```python
from build123d import *

# Parameters (mm, degrees)
SKETCH1_W           = 25.4
SKETCH1_H           = 12.7
BOSS_EXTRUDE1_DEPTH = 3.175
SKETCH2_W           = 6.4262
SKETCH2_H           = 3.175
BOSS_EXTRUDE2_DEPTH = 3.175
CUT_EXTRUDE1_DEPTH  = 3.175


with BuildPart() as part:
    # Sketch1 → Boss-Extrude1 (new body)
    with BuildSketch(Plane(origin=(0, 0, 0), x_dir=(1, 0, 0), z_dir=(0, 1, 0))):
        Rectangle(SKETCH1_W, SKETCH1_H)
    extrude(amount=BOSS_EXTRUDE1_DEPTH)

    # Sketch2 → Boss-Extrude2 (add)
    with BuildSketch(Plane.XY.offset(6.35)):
        with Locations((9.4869, 1.5875)):
            Rectangle(SKETCH2_W, SKETCH2_H)
        with Locations((-3.2893, 1.5875)):
            Rectangle(SKETCH2_W, SKETCH2_H)
    boss_extrude2 = extrude(amount=BOSS_EXTRUDE2_DEPTH)

    # Mirror1: Boss-Extrude2 across plane
    add(boss_extrude2.mirror(Plane.XY))

    # Sketch3 → Cut-Extrude1 (cut)
    with BuildSketch(Plane(origin=(0, 3.175, 0), x_dir=(1, 0, 0), z_dir=(0, 1, 0))):
        Polygon((-6.5024, -6.35), (-12.7, 6.35), (-12.7, -6.35), align=None)
    extrude(amount=-CUT_EXTRUDE1_DEPTH, mode=Mode.SUBTRACT)


solid = part.part
```
Design review of the part built by this model. Coordinates are the model's own, in mm. A direction names the side the tool comes from. Coordinates: 2 decimals unless noted, no trailing zeros. Order: outer loops, then holes, each group sorted by start corner. A loop starts at its lowest first (then second) coordinate and runs counter-clockwise, first axis right, second up. Notation, with made-up numbers: (-4.5, 63.5) - (5.5, 63.5) arc R27 ccw to (5.5, 98.5) - close; hole circle Ø7 at (73, -37). An arc over 180 degrees is marked (long way). Answer in a Markdown table with one row per item.
(1) Consider section C-C on z = -0.75. State the section outline as (x, y) points (3 decimals), plus the area to 3 significant figures.
Checked values:
| item | result |
|---|---|
| outline | (-9.967, 0) - (12.7, 0) - (12.7, 3.175) - (-9.967, 3.175) - close |
| area | 72.0 mm^2 |
(2) Consider section A-A on z = -7.25. State the section outline as (x, y) points (3 decimals), plus the area to 3 significant figures.
Checked values:
| item | result |
|---|---|
| outline | (-6.502, 0) - (-0.076, 0) - (-0.076, 3.175) - (-6.502, 3.175) - close; (6.274, 0) - (12.7, 0) - (12.7, 3.175) - (6.274, 3.175) - close |
| area | 40.8 mm^2 |
(3) Consider section B-B on y = 2.8. State the section outline as (x, z) points (3 decimals), plus the area to 3 significant figures.
Checked values:
| item | result |
|---|---|
| outline | (-12.7, -6.35) - (-6.502, -6.35) - (-6.502, -9.525) - (-0.076, -9.525) - (-0.076, -6.35) - (6.274, -6.35) - (6.274, -9.525) - (12.7, -9.525) - (12.7, 9.525) - (6.274, 9.525) - (6.274, 6.35) - (-0.076, 6.35) - (-0.076, 9.525) - (-6.502, 9.525) - (-6.502, 6.35) - close |
| area | 365 mm^2 |
(4) For faces 4 (the flat face through (3, 0, 0)), 5 (the flat face through (6.274, 2, -8)), 6 (the flat face through (-0.076, 2, 8)), 7 (the flat face through (-6.502, 2, -8)), list the 3-axis set-ups (+Z, -Z, +X, -X, +Y, -Y) from which the entire face can be reached by the end or side of a thin tool; tool diameter is ignored.
Checked values:
| item | result |
|---|---|
| face 4 | +Z, -Z, +X, -X, -Y |
| face 5 | -Z, +Y, -Y |
| face 6 | +Z, +Y, -Y |
| face 7 | -Z, -X, +Y, -Y |
(5) The part is to be moulded in two halves that separate along X. For faces 1 (the flat face through (-6.502, 2, 8)), 2 (the flat face through (3, 2, 6.35)), 3 (the flat face through (3, 3.175, 0)), say which applies: released by +X, released by -X, zero draft, split by the parting line, or undercut.
Checked values:
| item | result |
|---|---|
| face 1 | released by -X |
| face 2 | undercut |
| face 3 | zero draft |
(6) Wall thickness on line 1 along X through (y, z) = (0.95, 7.75); line 2 along Z through (x, y) = (3.75, 2.95); line 3 along Z through (x, y) = (-10, 1.7): over which ranges is each line inside the solid? List them lowest first. Write a range as from..to.
Checked values:
| item | result |
|---|---|
| line 1 | -6.5..-0.08, 6.27..12.7 |
| line 2 | -6.35..6.35 |
| line 3 | -6.35..-0.82 |
(7) Consider section D-D on z = -4.75. State the section outline as (x, y) points (3 decimals).
Checked values:
| item | result |
|---|---|
| outline | (-11.919, 0) - (12.7, 0) - (12.7, 3.175) - (-11.919, 3.175) - close |
(8) Clearance check with flat-ended pins moving along their axes: pin 1 (1.6 mm diameter, centred on x = 3, y = 2, fed in from -Z); pin 2 (1 mm diameter, centred on y = 1, z = 7, fed in from -X); pin 3 (1.5 mm diameter, centred on y = 2, z = -4.5, fed in from -X). State where each tip first meets the part, or that it passes through.
Checked values:
| item | result |
|---|---|
| pin 1 | z = -6.35 |
| pin 2 | x = -6.5 |
| pin 3 | x = -12.16 |
